from build123d import *

# Parameters (mm, degrees)
SZKIC1_R                    = 120
DODANIE_WYCI_GNI_CIE1_DEPTH = 30
SZKIC2_R                    = 100
WYTNIJ_WYCI_GNI_CIE1_DEPTH  = 20
SZKIC3_R                    = 4.5
WYTNIJ_WYCI_GNI_CIE2_DEPTH  = 171.880074906
SZKIC4_R                    = 25
WYTNIJ_WYCI_GNI_CIE3_DEPTH  = 171.880074906
SZKIC5_R                    = 85
SZKIC5_R_2                  = 80
DODANIE_WYCI_GNI_CIE2_DEPTH = 10
WYTNIJ_WYCI_GNI_CIE4_START  = -30
SZKIC6_R                    = 120
SZKIC6_R_2                  = 110
WYTNIJ_WYCI_GNI_CIE4_DEPTH  = 20


with BuildPart() as part:
    # Szkic1 → Dodanie-wyciągnięcie1 (new body)
    with BuildSketch(Plane(origin=(0, 0, 0), x_dir=(0, 0, -1), z_dir=(1, 0, 0))):
        Circle(SZKIC1_R)
    extrude(amount=DODANIE_WYCI_GNI_CIE1_DEPTH)

    # Szkic2 → Wytnij-wyciągnięcie1 (cut)
    with BuildSketch(Plane(origin=(30, 0, 0), x_dir=(0, 0, -1), z_dir=(1, 0, 0))):
        Circle(SZKIC2_R)
    extrude(amount=-WYTNIJ_WYCI_GNI_CIE1_DEPTH, mode=Mode.SUBTRACT)

    # Szkic3 → Wytnij-wyciągnięcie2 (cut, through all)
    with BuildSketch(Plane(origin=(10, 0, 0), x_dir=(0, 0, -1), z_dir=(1, 0, 0))):
        with Locations((0, 38.1)):
            Circle(SZKIC3_R)
        with Locations((26.940768363, 26.940768363)):
            Circle(SZKIC3_R)
        with Locations((38.1, 0)):
            Circle(SZKIC3_R)
        with Locations((26.940768363, -26.940768363)):
            Circle(SZKIC3_R)
        with Locations((0, -38.1)):
            Circle(SZKIC3_R)
        with Locations((-26.940768363, -26.940768363)):
            Circle(SZKIC3_R)
        with Locations((-38.1, 0)):
            Circle(SZKIC3_R)
        with Locations((-26.940768363, 26.940768363)):
            Circle(SZKIC3_R)
    extrude(amount=-WYTNIJ_WYCI_GNI_CIE2_DEPTH, mode=Mode.SUBTRACT)

    # Szkic4 → Wytnij-wyciągnięcie3 (cut, through all)
    with BuildSketch(Plane(origin=(10, 0, 0), x_dir=(0, 0, -1), z_dir=(1, 0, 0))):
        Circle(SZKIC4_R)
    extrude(amount=-WYTNIJ_WYCI_GNI_CIE3_DEPTH, mode=Mode.SUBTRACT)

    # Szkic5 → Dodanie-wyciągnięcie2 (add)
    with BuildSketch(Plane(origin=(10, 0, 0), x_dir=(0, 0, -1), z_dir=(1, 0, 0))):
        Circle(SZKIC5_R)
        Circle(SZKIC5_R_2, mode=Mode.SUBTRACT)
    extrude(amount=DODANIE_WYCI_GNI_CIE2_DEPTH)

    # Szkic6 → Wytnij-wyciągnięcie4 (cut)
    with BuildSketch(Plane(origin=(30, 0, 0), x_dir=(0, 0, -1), z_dir=(1, 0, 0)).offset(WYTNIJ_WYCI_GNI_CIE4_START)):
        Circle(SZKIC6_R)
        Circle(SZKIC6_R_2, mode=Mode.SUBTRACT)
    extrude(amount=WYTNIJ_WYCI_GNI_CIE4_DEPTH, mode=Mode.SUBTRACT)


solid = part.part
Model file for the job. Use its own axes, mm. A direction names the side the tool comes from. Give positions to 0.01 mm unless a question says otherwise; leave off trailing zeros. Order: outer loops, then holes, each group sorted by start corner. A loop starts at its lowest first (then second) coordinate and runs counter-clockwise, first axis right, second up. Notation, with made-up numbers: (-23.75, -28) - (20.25, -28) arc R20 cw to (20.25, 10) - close; hole circle Ø8 at (-20.75, 17). An arc over 180 degrees is marked (long way). One line per item, written item: value.
Item 1: Pin check, flat tips, straight feed: pin 1 Ø5 at (x, y) = (6.5, 59.5) entering from -Z; pin 2 Ø10 at (x, y) = (20, 91.5) entering from +Z; pin 3 Ø10 at (x, z) = (9, -81) entering from -Y. Stop position of each tip, or through.
Response values:
pin 1: z = -94.08
pin 2: z = 83.17
pin 3: y = -79.52
Item 2: Two-plate mould, pull along Z, no slides. Class faces 1 (the cylindrical face through (9.86, -107.384, 23.846)), 2 (the cylindrical face through (20.14, 30.04, -95.38)), 3 (the flat face through (20, -97, -53)): released by +Z, released by -Z, zero draft, split by the parting line, or undercut.
Response values:
face 1: split by the parting line
face 2: undercut
face 3: zero draft
Item 3: Slice it at A-A (z = 0). Give the number of separate pieces and of enclosed holes in the cut face, then the cut area to 3 significant figures.
Response values:
separate pieces: 4
enclosed holes: 0
area: 2,220 mm2
Item 4: Tool access for faces 4 (the flat face through (10, -17, 19)), 5 (the cylindrical face through (5.07, 33.71, 0.98)): list every direction of +Z, -Z, +X, -X, +Y, -Y with a clear straight run to the whole face (end or side of a thin tool).
Response values:
face 4: +X
face 5: +X, -X
Item 5: Slice it at C-C (x = 17). List the corners of the cut face in (y, z), then the cut area to 3 significant figures.
Response values:
outline: circle Ø220 at (0, 0); circle Ø170 at (0, 0); hole circle Ø200 at (0, 0); hole circle Ø160 at (0, 0)
area: 9,190 mm2
Item 6: Slice it at B-B (z = -38.1). List the corners of the cut face in (x, y).
Response values:
outline: (0, -103.19) - (20, -103.19) - (20, -113.79) - (30, -113.79) - (30, -92.46) - (10, -92.46) - (10, -75.98) - (20, -75.98) - (20, -70.34) - (10, -70.34) - (10, -4.5) - (0, -4.5) - close; (0, 4.5) - (10, 4.5) - (10, 70.34) - (20, 70.34) - (20, 75.98) - (10, 75.98) - (10, 92.46) - (30, 92.46) - (30, 113.79) - (20, 113.79) - (20, 103.19) - (0, 103.19) - close
Item 7: Wall check: line 1 (Y direction, x = 17, z = 0); line 2 (Y direction, x = 19.75, z = 26.5); line 3 (Z direction, x = 12.75, y = 69.5). Give the ranges that are in metal, low to high.
Response values:
line 1: -110 to -100, -85 to -80, 80 to 85, 100 to 110
line 2: -106.76 to -96.42, -80.76 to -75.48, 75.48 to 80.76, 96.42 to 106.76
line 3: -85.26 to -71.9, -48.94 to -39.62, 39.62 to 48.94, 71.9 to 85.26
